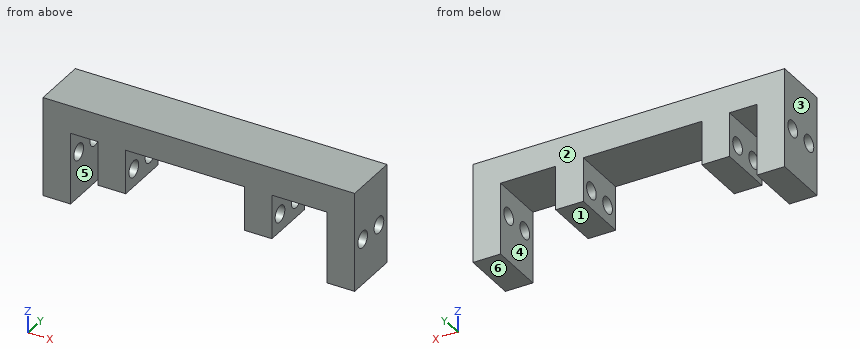
Autodesk Inventor part; units mm, degrees
ref_plane "YZ Plane" through (0, 0, 0) normal (1, 0, 0) x (0, 1, 0)
ref_plane "XZ Plane" through (0, 0, 0) normal (0, 1, 0) x (-1, 0, 0)
ref_plane "XY Plane" through (0, 0, 0) normal (0, 0, 1) x (1, 0, 0)
sketch "Sketch1" plane through (0, 0, 0) normal (0, 1, 0) x (-1, 0, 0)
  line L0 (-6.122, -0.5654) -> (40.378, -0.5654)
  line L1 (40.378, -0.5654) -> (40.378, -5.5654)
  line L2 (40.378, -5.5654) -> (-6.122, -5.5654)
  line L3 (-6.122, -5.5654) -> (-6.122, -0.5654)
  line L4 (40.378, -0.5654) -> (45.378, -0.5654)
  line L5 (45.378, -0.5654) -> (45.378, -5.5654)
  line L6 (45.378, -5.5654) -> (40.378, -5.5654)
  line L7 (45.378, -5.5654) -> (45.378, -13.5654)
  line L8 (45.378, -13.5654) -> (40.378, -13.5654)
  line L9 (40.378, -13.5654) -> (40.378, -5.5654)
  line L10 (35.378, -13.5654) -> (35.378, -5.5654)
  line L11 (35.378, -13.5654) -> (30.378, -13.5654)
  line L12 (30.378, -13.5654) -> (30.378, -5.5654)
  line L13 (-6.122, -0.5654) -> (-11.122, -0.5654)
  line L14 (-11.122, -0.5654) -> (-11.122, -5.5654)
  line L15 (-11.122, -5.5654) -> (-6.122, -5.5654)
  line L16 (-11.122, -5.5654) -> (-11.122, -13.5654)
  line L17 (-11.122, -13.5654) -> (-6.122, -13.5654)
  line L18 (-6.122, -5.5654) -> (3.878, -5.5654)
  line L19 (3.878, -5.5654) -> (3.878, -13.5654)
  line L20 (3.878, -13.5654) -> (8.878, -13.5654)
  line L21 (8.878, -13.5654) -> (8.878, -5.5654)
  line L22 (-6.122, -5.5654) -> (-6.122, -13.5654)
  point P0 (0, 0)
  dimension "d0" = 46.5
  dimension "d1" = 5
  dimension "d2" = 5
  dimension "d3" = 8
  dimension "d4" = 5
  dimension "d5" = 5
  dimension "d6" = 5
  dimension "d7" = 8
  dimension "d8" = 10
  dimension "d9" = 5
extrude "Extrusion1" add sketch "Sketch1" along normal blind 10
sketch "Sketch2" plane through (-45.378, 0, -13.5654) normal (-1, 0, 0) x (0, 0, 1)
  line L0 (0, 10) -> (13, 10)
  line L1 (13, 10) -> (0, 10)
  line L2 (0, 10) -> (6.5, 10)
  line L3 (0, 0) -> (8, 0)
  line L4 (6.5, 0) -> (6.5, 10)
  line L5 (6.5, 5) -> (0, 5)
  line L6 (0, 5) -> (3.25, 5)
  line L7 (3.25, 0) -> (3.25, 5)
  line L8 (3.25, 10) -> (3.25, 5)
  circle A0 centre (3.25, 7.5) radius 1.5
  circle A1 centre (3.25, 2.5) radius 1.5
  point P0 (13.5654, 0)
  dimension "d12" = 3
  dimension "d13" = 3
extrude "Extrusion2" cut sketch "Sketch2" against normal blind 60 contours A0 L8 | L8 A0 | A1 L7 | L7 A1
thread "Thread1"
thread "Thread2"
thread "Thread3"
thread "Thread4"
thread "Thread5"
thread "Thread6"
thread "Thread7"
thread "Thread8"
sketch "Sketch3" plane through (-40.378, 0, -13.5654) normal (0, 0, -1) x (-1, 0, 0)
  line L0 (5, 10) -> (-51.5, 10)
  line L1 (5, 0) -> (5, 10)
  line L2 (0.1606, 10) -> (5, 10)
  line L3 (5, 10) -> (5, 0)
  line L4 (5, 0) -> (0.1606, 0)
  line L5 (0.1606, 0) -> (0.1606, 10)
  line L6 (-10, 0) -> (-10, 10)
  line L7 (-5, 0) -> (-5, 10)
  line L8 (-10, 10) -> (-5, 10)
  line L9 (-5, 10) -> (-5, 0)
  line L10 (-5, 0) -> (-10, 0)
  line L11 (-10, 0) -> (-10, 10)
  line L12 (-36.5, 0) -> (-36.5, 10)
  line L13 (-31.5, 0) -> (-31.5, 10)
  line L14 (-36.5, 10) -> (-31.5, 10)
  line L15 (-31.5, 10) -> (-31.5, 0)
  line L16 (-31.5, 0) -> (-36.5, 0)
  line L17 (-36.5, 0) -> (-36.5, 10)
  line L18 (-46.5, 0) -> (-46.5, 10)
  line L19 (-51.5, 0) -> (-51.5, 10)
  line L20 (-46.5, 0) -> (-51.5, 0)
  line L21 (-51.5, 0) -> (-51.5, 10)
  line L22 (-51.5, 10) -> (-46.5, 10)
  line L23 (-46.5, 10) -> (-46.5, 0)
  line L24 (0, 10) -> (5, 10)
  line L25 (5, 10) -> (5, 0)
  line L26 (5, 0) -> (0, 0)
  line L27 (0, 0) -> (0, 10)
  point P0 (-40.378, 0)
extrude "Extrusion3" add sketch "Sketch3" along normal blind 5 contours L1 L4 L5 L0 | L18 L20 L19 L0 | L5 L26 L27 L0
sketch "Sketch4" plane through (0, 10, 0) normal (0, 1, 0) x (1, 0, 0)
  point P0 (0, 0)
properties part number "soporte"
Build history of the part. All positions in model axes, mm. Face numbers are marked on the shaded views. A direction names the side the tool comes from. Round coordinates to 2 decimals unless told otherwise and drop trailing zeros. Loops run counter-clockwise (first coordinate to the right, second up) from the corner with the lowest first, then second, coordinate; pieces in that order, holes last. Notation, with made-up numbers: M -22.5,50 L 24.5,50 A26 ccw 24.5,65 Z; hole C 57,75.25 d2. An arc over 180 degrees is marked long. Answer as CSV lines item,"result".
1. Two-plate mould, pull along X, no slides. Class the marked faces 1, 2, 3 and 4: released by +X, released by -X, zero draft, split by the parting line, or undercut.
Resolved:
face 1,"undercut"
face 2,"zero draft"
face 3,"released by -X"
face 4,"undercut"
2. Flat gauge pins, fed straight in: P1, Ø5, axis at y = 7.5, z = -10.32, coming from the +X side; P2, Ø5.5, axis at x = -34, y = 2.5, coming from the -Z side; P3, Ø2.5, axis at y = 2.5, z = -10.32, coming from the +X side; P4, Ø3, axis at x = 0.5, y = 3, coming from the -Z side. Where does each tip first touch, or does it go through?
Resolved:
P1,"stops at x = 11.12"
P2,"stops at z = -13.57"
P3,"passes through"
P4,"stops at z = -5.57"
3. Wall check: probe 1 along X at (y, z) = (4.75, -8.5); probe 2 along Z at (x, y) = (-44.15, 2.5); probe 3 along X at (y, z) = (3.5, -13.75). Give the ranges that are in metal, low to high. Write a range as [from, to].
Resolved:
probe 1,"x = [-45.38, -40.38], [-35.38, -30.38], [-8.88, -3.88], [6.12, 11.12]"
probe 2,"z = [-18.57, -11.82], [-8.82, -0.57]"
probe 3,"x = [-45.38, -40.38], [6.12, 11.12]"
4. Cut at A-A on y = 2.5. Count the separate pieces of the cut face and the enclosed holes in it, then the cut area to 4 significant figures.
Resolved:
separate pieces,"5"
enclosed holes,"0"
area,"432.5 mm²"
5. Cut at D-D on x = -25. Write the cut outline in (y, z), then the cut area to 3 significant figures.
Resolved:
outline,"M 0,-5.57 L 10,-5.57 L 10,-0.57 L 0,-0.57 Z"
area,"50.0 mm²"
6. Cut at B-B on x = -41. Write the cut outline in (y, z).
Resolved:
outline,"M 0,-18.57 L 10,-18.57 L 10,-0.57 L 0,-0.57 Z; hole C 2.5,-10.32 d3; hole C 7.5,-10.32 d3"
7. 3-axis set-ups, long thin cutter, end or side, ignore diameter. For the marked faces 5 and 6: which of +Z, -Z, +X, -X, +Y, -Y reach the whole face in a straight line?
Resolved:
face 5,"-Z, +Y, -Y"
face 6,"-Z, +X, -X, +Y, -Y"
